The listing builds one solid part. Answer for the finished solid, in the listing's coordinates (mm). A direction names the side the tool comes from. Round coordinates to 2 decimals unless told otherwise and drop trailing zeros. Write each loop counter-clockwise with the first axis right and the second up, starting at its lowest first coordinate (ties: lowest second). Pieces come first, ordered by that corner, then holes.
from build123d import *

# Parameters (mm, degrees)
SKETCH002_W      = 160.74
SKETCH002_H      = 210
SKETCH002_R      = 1.6
EXTRUDE002_DEPTH = 1.6
SKETCH007_W      = 28
SKETCH007_H      = 6
EXTRUDE007_DEPTH = 10


with BuildPart() as extrude002:
    # Sketch002 → Extrude002 (new body)
    with BuildSketch(Plane.XY.offset(8)):
        with Locations((80.37, 105)):
            Rectangle(SKETCH002_W, SKETCH002_H)
        with Locations((6, 204)):
            Circle(SKETCH002_R, mode=Mode.SUBTRACT)
        with Locations((154.74, 204)):
            Circle(SKETCH002_R, mode=Mode.SUBTRACT)
        with Locations((154.74, 6)):
            Circle(SKETCH002_R, mode=Mode.SUBTRACT)
        with Locations((6, 6)):
            Circle(SKETCH002_R, mode=Mode.SUBTRACT)
    extrude(amount=EXTRUDE002_DEPTH)


with BuildPart() as obj1:
    # Sketch007 (on Face10 of Extrude002) → Extrude007 (new body)
    with BuildSketch(Plane.XY.offset(9.6)):
        with Locations((143.552, 99.603)):
            Rectangle(SKETCH007_W, SKETCH007_H)
        with Locations((143.552, 88.173)):
            Rectangle(SKETCH007_W, SKETCH007_H)
        with Locations((143.552, 76.743)):
            Rectangle(SKETCH007_W, SKETCH007_H)
    extrude(amount=EXTRUDE007_DEPTH)

    # Fusion002: union Extrude002
    add(extrude002.part)


solid = obj1.part
1. Section B-B on x = 118 is taken. Determine the outline of the cut face in (y, z), plus the area to 3 significant figures.
Geometry says:
outline: (0, 8) - (210, 8) - (210, 9.6) - (0, 9.6) - close
area: 336 mm2
2. Straight lines are drawn through the part: line 1 along X through (y, z) = (204, 9.2); line 2 along Y through (x, z) = (154.74, 9.05); line 3 along Y through (x, z) = (141, 18.5). For each, find the intervals that lie inside material, in ascending order.
Geometry says:
line 1: x = 0 to 4.4, 7.6 to 153.14, 156.34 to 160.74
line 2: y = 0 to 4.4, 7.6 to 202.4, 205.6 to 210
line 3: y = 73.74 to 79.74, 85.17 to 91.17, 96.6 to 102.6
3. Section C-C on y = 118.5 is taken. Determine the outline of the cut face in (x, z), plus the area to 3 significant figures.
Geometry says:
outline: (0, 8) - (160.74, 8) - (160.74, 9.6) - (0, 9.6) - close
area: 257 mm2
4. A tool of negligible diameter and unlimited length cuts with its end or side. For faces 1 (the face through (129.552, 77, 15)), 2 (the face through (157.552, 100, 15)), 3 (the face through (143, 73.743, 15)), from which of +Z, -Z, +X, -X, +Y, -Y can it reach the whole face along a straight path? Write none if from no direction.
Geometry says:
face 1: +Z, -X, +Y, -Y
face 2: +Z, +X, +Y, -Y
face 3: +Z, +X, -X, -Y
5. Given pin 1 (3 mm diameter, centred on y = 76.5, z = 12, fed in from +X); pin 2 (5 mm diameter, centred on x = 139.5, z = 12.5, fed in from -Y); pin 3 (1.8 mm diameter, centred on y = 87.5, z = 16, fed in from -X); pin 4 (1.5 mm diameter, centred on x = 128.5, z = 14, fed in from -Y), each flat-ended and moving along its own axis, determine where each tip first touches the part or whether it passes through.
Geometry says:
pin 1: stops at x = 157.55
pin 2: stops at y = 73.74
pin 3: stops at x = 129.55
pin 4: passes through
6. Section A-A on z = 12.25 is taken. Determine the outline of the cut face in (x, y), plus the area to 3 significant figures.
Geometry says:
outline: (129.55, 73.74) - (157.55, 73.74) - (157.55, 79.74) - (129.55, 79.74) - close; (129.55, 85.17) - (157.55, 85.17) - (157.55, 91.17) - (129.55, 91.17) - close; (129.55, 96.6) - (157.55, 96.6) - (157.55, 102.6) - (129.55, 102.6) - close
area: 504 mm2
